Model file for the job. Use its own axes, mm. Coordinates: 2 decimals unless noted, no trailing zeros. Loops run counter-clockwise (first coordinate to the right, second up) from the corner with the lowest first, then second, coordinate; pieces in that order, holes last. Notation, with made-up numbers: M 62.25,-13 L 120.25,-13 A24 ccw 120.25,15 Z; hole C 2.5,44 d1. An arc over 180 degrees is marked long. Write item = value, one per line. Start each with the question number.
from build123d import *

# Parameters (mm, degrees)
F0_R     = 5
F1_DEPTH = 8
F2_SIZE  = 1


with BuildPart() as f1:
    # F0 (on Top) → F1 (new body)
    with BuildSketch(Plane.XY):
        Polygon((0, -9.814955), (8.5, -4.907477), (8.5, 4.907477), (0, 9.814955), (-8.5, 4.907477), (-8.5, -4.907477), align=None)
        Circle(F0_R, mode=Mode.SUBTRACT)
    extrude(amount=F1_DEPTH)

    # F2
    f2_edges = [f1.edges().sort_by_distance(p)[0] for p in [
        (-5, 0, 8),
        (-5, 0, 0),
    ]]
    chamfer(f2_edges, length=F2_SIZE)

    # F3 (on Front) → F4 (revolve, cut)
    with BuildSketch(Plane.XZ):
        Polygon((18.032537, 8), (8.5, 8), (18.032537, 2.496387), align=None)
    revolve(axis=Axis((0, 0, 4), (0, 0, -1)), mode=Mode.SUBTRACT)


solid = f1.part
Item 1: Cut at A-A (z = 3). Give the cut face in (x, y), plus the area to 3 significant figures.
Item 2: Probe L1, parallel to X at y = -3.5, z = 0.75; L2, parallel to Y at x = 0.5, z = 6; L3, parallel to X at y = 0.5, z = 2.5. List the from-to ranges inside material, lowest first.
Item 3: Pull direction Y, two halves, no side cores. Call faces 1 (the flat face through (-4.19, 7.396, 3.944)), 2 (the cylindrical face through (-1.08, -4.88, 3.96)), 3 (the flat face through (-8.5, 0, 4)), 4 (the conical face through (7.649, -4.391, 7.815)): +Y half, -Y half, draft (parallel to the pull), parting line (faces both ways), or undercut.
Reported:
q1.outline = M -8.5,-4.91 L 0,-9.81 L 8.5,-4.91 L 8.5,4.91 L 0,9.81 L -8.5,4.91 Z; hole C 0,0 d10
q1.area = 172 mm^2
q2.L1 = -8.5 to -3.91, 3.91 to 8.5
q2.L2 = -9.53 to -4.97, 4.97 to 9.53
q2.L3 = -8.5 to -4.97, 4.97 to 8.5
q3.face_1 = +Y half
q3.face_2 = undercut
q3.face_3 = draft
q3.face_4 = -Y half
